Autodesk Inventor part; units mm, degrees
ref_plane "YZ Plane" through (0, 0, 0) normal (1, 0, 0) x (0, 1, 0)
ref_plane "XZ Plane" through (0, 0, 0) normal (0, 1, 0) x (-1, 0, 0)
ref_plane "XY Plane" through (0, 0, 0) normal (0, 0, 1) x (1, 0, 0)
sketch "スケッチ1" plane through (0, 0, 0) normal (0, 1, 0) x (-1, 0, 0)
  line L0 (0, 0) -> (-90, 0)
  line L1 (-90, 0) -> (-90, 50)
  line L2 (0, 50) -> (0, 0)
  line L3 (0, 0) -> (-5, 0)
  line L4 (-5, 0) -> (-5, 50)
  line L5 (-5, 0) -> (-90, 0)
  line L6 (-90, 0) -> (-85, 0)
  line L7 (-85, 0) -> (-85, 50)
  arc A0 (-85, 50) -> (-5, 50) centre (-45, 50) ccw
  line L8 (0, 0) -> (0, 10)
  line L9 (0, 10) -> (-90, 10)
  circle A1 centre (-45, 50) radius 45
  line L10 (-90, 5) -> (0, 5)
  line L11 (-90, 50) -> (-85, 50)
  line L12 (-5, 50) -> (0, 50)
  line L13 (0, 0) -> (-90, 0)
  line L14 (-90, 0) -> (-90, 5)
  line L15 (-90, 5) -> (0, 5)
  line L16 (0, 5) -> (0, 0)
  dimension "d0" = 90
  dimension "d1" = 50
  dimension "d2" = 5
  dimension "d3" = 85
  dimension "d4" = 5
  dimension "d5" = 80
  dimension "d6" = 10
  dimension "d7" = 90
extrude "押し出し1" add sketch "スケッチ1" along normal blind 230 contours L0 L4 L10 L2 | L0 L7 L10 L4 | L10 L4 L9 L2 | L0 L1 L10 L7 | L10 A1 L9 L4 | L9 L4 A1 L2 | L10 L1 L9 L7 | L7 L9 A1 L10 | L9 A1 L4 | A1 L9 | A1 L4 L12 | L9 L1 A1 L7 | L7 A1 L9 | A1 L9 A0 L4 | A1 L7 A0 L9 | L11 L7 A1
sketch "スケッチ2" plane through (0, 0, 0) normal (0, -1, 0) x (1, 0, 0)
  line L0 (0, 0) -> (0, 50)
  line L1 (90, 0) -> (0, 0)
  line L2 (90, 50) -> (90, 0)
  line L3 (85, 50) -> (90, 50)
  arc A0 (5, 50) -> (85, 50) centre (45, 50) ccw
  line L4 (0, 50) -> (5, 50)
  arc A1 (5, 23.467) -> (85, 23.467) centre (45, 50) ccw
  line L5 (0, 5) -> (90, 5)
  line L6 (5, 23.467) -> (5, 5)
  line L7 (85, 23.467) -> (85, 5)
  dimension "d29" = 48
extrude "押し出し2" cut sketch "スケッチ2" against normal blind 225 contours L6 A1 L5 | L5 A1 L7
sketch "スケッチ3" plane through (0, 230, 0) normal (0, 1, 0) x (1, 0, 0)
  arc A0 (85, -50) -> (5, -50) centre (45, -50) ccw
  line L0 (90, -50) -> (90, 0)
  line L1 (0, -50) -> (5, -50)
  arc A1 (85, -50) -> (5, -50) centre (45, -50) ccw
  line L2 (5, -50) -> (85, -50)
extrude "押し出し3" add sketch "スケッチ3" against normal blind 5
sketch "スケッチ4" plane through (90, 0, 50) normal (1, 0, 0) x (0, 0, -1)
  line L0 (0, 0) -> (50, 0)
  line L1 (0, 0) -> (0, 230)
  line L2 (25, 0) -> (25, 65)
  line L3 (25, 65) -> (25, 75)
  line L4 (25, 75) -> (25, 215)
  line L5 (25, 215) -> (25, 225)
  line L6 (0, 65) -> (40, 65)
  line L7 (40, 65) -> (40, 75)
  line L8 (40, 75) -> (0, 75)
  line L9 (0, 75) -> (0, 65)
  line L10 (0, 215) -> (40, 215)
  line L11 (40, 215) -> (40, 225)
  line L12 (40, 225) -> (0, 225)
  line L13 (0, 225) -> (0, 215)
  dimension "d16" = 65
  dimension "d17" = 10
  dimension "d18" = 140
  dimension "d19" = 10
  dimension "d20" = 40
extrude "押し出し4" cut sketch "スケッチ4" against normal blind 90 contours L1 L8 L3 L6 | L3 L8 L7 L6 | L1 L12 L5 L10 | L5 L12 L11 L10
sketch "スケッチ6" plane through (90, 0, 50) normal (1, 0, 0) x (0, 0, -1)
  line L0 (0, 230) -> (50, 230)
  line L1 (50, 230) -> (37.5, 251.6506)
  line L2 (50, 230) -> (110, 230) construction
  line L3 (0, 230) -> (37.5, 251.6506)
  line L4 (0, 230) -> (43.3013, 230) construction
  dimension "d32" = 120
  dimension "d33" = 30
extrude "押し出し6" add sketch "スケッチ6" against normal blind 90
sketch "スケッチ9" plane through (0, 0, 0) normal (-1, 0, 0) x (0, 0, 1)
  line L0 (10, 225) -> (50, 225)
  line L1 (50, 225) -> (50, 230)
  line L2 (50, 230) -> (12.5, 251.6506)
  line L3 (12.5, 251.6506) -> (0, 230)
  line L4 (0, 0) -> (0, 230)
  line L5 (0, 0) -> (50, 0)
  line L6 (50, 0) -> (50, 65)
  line L7 (50, 65) -> (10, 65)
  line L8 (10, 65) -> (10, 75)
  line L9 (10, 75) -> (50, 75)
  line L10 (50, 75) -> (50, 215)
  line L11 (50, 215) -> (10, 215)
  line L12 (10, 215) -> (10, 225)
  line L13 (12.5, 251.6506) -> (0, 230)
  line L14 (0, 230) -> (-132.7906, 0)
  line L15 (0, 145) -> (-49.0748, 145)
  line L16 (0, 115) -> (-66.3953, 115)
  dimension "d45" = 30
sketch "スケッチ10" plane through (0, 0, 0) normal (-1, 0, 0) x (0, 0, 1)
  line L0 (10, 225) -> (50, 225)
  line L1 (50, 225) -> (50, 230)
  line L2 (50, 230) -> (12.5, 251.6506)
  line L3 (12.5, 251.6506) -> (0, 230)
  line L4 (0, 0) -> (0, 230)
  line L5 (0, 0) -> (50, 0)
  line L6 (50, 0) -> (50, 65)
  line L7 (50, 65) -> (10, 65)
  line L8 (10, 65) -> (10, 75)
  line L9 (10, 75) -> (50, 75)
  line L10 (50, 75) -> (50, 215)
  line L11 (50, 215) -> (10, 215)
  line L12 (10, 215) -> (10, 225)
  line L13 (12.5, 251.6506) -> (-87.5, 78.4456)
  line L14 (-87.5, 78.4456) -> (50, 0)
sketch "スケッチ11" plane through (90, 230, 0) normal (0, 0.5, -0.866) x (-1, 0, 0)
  line L0 (0, 25) -> (90, 25)
  line L1 (45, 25) -> (45, 15)
  line L2 (45, 15) -> (60, 15)
  line L3 (60, 15) -> (30, 15)
  point P0 (90, -199.1858)
  dimension "d49" = 10
  dimension "d50" = 15
  dimension "d51" = 30
hole "穴1" at (45, 242.9904, 7.5) at (30, 242.9904, 7.5) at (60, 242.9904, 7.5) direction (0, -0.5, 0.866) diameter 2.5 depth 8 tip angle 118
sketch "スケッチ12" plane through (90, 0, 50) normal (1, 0, 0) x (0, 0, -1)
  line L0 (50, 0) -> (50, 230)
  line L1 (40, 225) -> (40, 215)
  line L2 (0, 215) -> (0, 75)
  line L3 (0, 145) -> (50, 145)
  line L4 (32.5, 175) -> (17.5, 175)
  line L5 (17.5, 175) -> (17.5, 115)
  line L6 (17.5, 115) -> (32.5, 115)
  line L7 (32.5, 115) -> (32.5, 175)
  line L8 (32.5, 175) -> (17.5, 115) construction
  line L9 (17.5, 175) -> (32.5, 115) construction
  line L10 (17.5, 145) -> (32.5, 145)
  line L11 (32.5, 145) -> (32.5, 115)
  line L12 (32.5, 115) -> (17.5, 115)
  line L13 (17.5, 115) -> (17.5, 145)
  point P0 (25, 145)
  dimension "d59" = 15
  dimension "d60" = 60
extrude "押し出し8" cut sketch "スケッチ12" against normal blind 2.5 contours L3 L7 L6 L5
sketch "スケッチ13" plane through (0, 0, 0) normal (-1, 0, 0) x (0, 0, 1)
  line L0 (0, 0) -> (0, 230)
  line L1 (50, 75) -> (50, 215)
  line L2 (50, 145) -> (0, 145)
  line L3 (17.5, 175) -> (32.5, 175)
  line L4 (32.5, 175) -> (32.5, 115)
  line L5 (32.5, 115) -> (17.5, 115)
  line L6 (17.5, 115) -> (17.5, 175)
  line L7 (17.5, 175) -> (32.5, 115) construction
  line L8 (32.5, 175) -> (17.5, 115) construction
  line L9 (17.5, 145) -> (32.5, 145)
  line L10 (32.5, 145) -> (32.5, 115)
  line L11 (32.5, 115) -> (17.5, 115)
  line L12 (17.5, 115) -> (17.5, 145)
  point P0 (25, 145)
  dimension "d63" = 15
  dimension "d64" = 60
extrude "押し出し9" cut sketch "スケッチ13" against normal blind 2.5 contours L4 L5 L6 L2
sketch "スケッチ14" plane through (90, 0, 0) normal (0, 0, -1) x (-1, 0, 0)
  line L0 (90, 0) -> (90, 230)
  line L1 (0, 0) -> (0, 230)
  line L2 (0, 145) -> (90, 145)
  line L3 (37.5, 175) -> (52.5, 175)
  line L4 (52.5, 175) -> (52.5, 115)
  line L5 (52.5, 115) -> (37.5, 115)
  line L6 (37.5, 115) -> (37.5, 175)
  line L7 (37.5, 175) -> (52.5, 115) construction
  line L8 (52.5, 175) -> (37.5, 115) construction
  line L9 (37.5, 145) -> (52.5, 145)
  line L10 (52.5, 145) -> (52.5, 175)
  line L11 (52.5, 175) -> (37.5, 175)
  line L12 (37.5, 175) -> (37.5, 145)
  point P0 (45, 145)
  dimension "d67" = 15
  dimension "d70" = 30
extrude "押し出し10" cut sketch "スケッチ14" against normal blind 2.5 contours L6 L3 L4 L2
sketch "スケッチ16" plane through (90, 0, 0) normal (0, 0, -1) x (-1, 0, 0)
  line L0 (52.5, 175) -> (52.5, 145)
  line L1 (52.5, 145) -> (37.5, 145)
  line L2 (37.5, 145) -> (37.5, 175)
  line L3 (90, 0) -> (90, 230)
  line L4 (0, 0) -> (0, 230)
  line L5 (0, 145) -> (90, 145)
  line L6 (0, 160) -> (37.5, 160)
  line L7 (52.5, 160) -> (90, 160)
  line L8 (18.75, 160) -> (18.75, 145)
  line L9 (71.25, 145) -> (71.25, 160)
  line L10 (11.25, 175) -> (26.25, 175)
  line L11 (26.25, 175) -> (26.25, 115)
  line L12 (26.25, 115) -> (11.25, 115)
  line L13 (11.25, 115) -> (11.25, 175)
  line L14 (11.25, 175) -> (26.25, 115) construction
  line L15 (26.25, 175) -> (11.25, 115) construction
  line L16 (11.25, 115) -> (26.25, 115)
  line L17 (26.25, 115) -> (26.25, 175)
  line L18 (26.25, 175) -> (11.25, 175)
  line L19 (11.25, 175) -> (11.25, 115)
  line L20 (45, 145) -> (45, 125)
  line L21 (78.75, 175) -> (63.75, 175)
  line L22 (63.75, 115) -> (78.75, 115)
  line L23 (78.75, 175) -> (78.75, 115)
  line L24 (63.75, 115) -> (63.75, 175)
  line L25 (63.75, 175) -> (78.75, 175)
  line L26 (78.75, 175) -> (78.75, 115)
  line L27 (78.75, 115) -> (63.75, 115)
  line L28 (63.75, 115) -> (63.75, 175)
  line L29 (11.25, 115) -> (26.25, 115)
  line L30 (26.25, 115) -> (26.25, 175)
  line L31 (26.25, 175) -> (11.25, 175)
  line L32 (11.25, 175) -> (11.25, 115)
  dimension "d71" = 15
  dimension "d72" = 60
  dimension "d73" = 20
extrude "押し出し11" cut sketch "スケッチ16" against normal blind 3 contours L24 L21 L23 L7 | L7 L9 L5 L24 | L5 L23 L22 L24 | L7 L23 L5 L9 | L11 L12 L13 L5 | L5 L8 L6 L11 | L6 L13 L10 L11 | L5 L13 L6 L8
sketch "スケッチ17" plane through (37.5, 145, 0) normal (0, 1, 0) x (1, 0, 0)
  line L0 (0, 0) -> (15, 0)
  line L1 (0, 0) -> (0, -2.5)
  line L2 (0, -2.5) -> (15, -2.5)
  line L3 (15, 0) -> (15, -2.5)
  line L4 (-57.7643, 16.522) -> (69.053, 16.522)
  line L5 (69.053, 16.522) -> (69.053, -65.9751)
  line L6 (69.053, -65.9751) -> (-57.7643, -65.9751)
  line L7 (-57.7643, -65.9751) -> (-57.7643, 16.522)
  point P0 (-37.5, 0)
properties part number "知能ロボコン発射台２．３" material "ABS プラスチック"
Design review of the part built by this model. Coordinates are the model's own, in mm. A direction names the side the tool comes from. Coordinates: 2 decimals unless noted, no trailing zeros. Order: outer loops, then holes, each group sorted by start corner. A loop starts at its lowest first (then second) coordinate and runs counter-clockwise, first axis right, second up.
Item 1: The part is to be moulded in two halves that separate along Y. For faces 5 (the flat face through (56, 0, 9)), 6 (the flat face through (44, 113, 0)), 7 (the flat face through (88, 220, 10)), say which applies: pulls with the +Y half, pulls with the -Y half, needs draft (parallel to the pull), parting line crosses it, or undercut.
Item 2: Take a section at B-B, the plane y = 71. Write out the cut boundary in (x, z), then the cut area to 3 significant figures.
Item 3: For line 1 (Y direction, x = 25, z = 12.5); line 2 (Y direction, x = 82, z = 22); line 3 (X direction, y = 152, z = 9), list the stretches that pass through material, from the lowest coordinate up.
Item 4: Take a section at C-C, the plane x = 67. Write out the cut boundary in (y, z), then the cut area to 3 significant figures.
Item 5: For pin 1 Ø12 at (x, z) = (27, 27) entering from +Y; pin 2 Ø1.5 at (x, y) = (87.5, 219.5) entering from +Z; pin 3 Ø1.5 at (x, y) = (68.5, 147.5) entering from +Z, all flat-tipped, find the tip position at first contact; note any pin that passes through.
Item 6: Take a section at A-A, the plane y = 104. Write out the cut boundary in (x, z).
Item 7: For faces 1 (the flat face through (87.5, 130, 25)), 2 (the cylindrical face through (44.16, 240.16, 10.55)), 3 (the flat face through (19, 145, 3)), 4 (the flat face through (9, 215, 24)), list the 3-axis set-ups (+Z, -Z, +X, -X, +Y, -Y) from which the entire face can be reached by the end or side of a thin tool; tool diameter is ignored.
The answers:
1. face 5: pulls with the -Y half
1. face 6: needs draft
1. face 7: undercut
2. outline: (0, 0) - (90, 0) - (90, 10) - (85, 10) - (85, 5) - (61.7, 5) arc R48 ccw to (71.53, 10) - (18.47, 10) arc R48 ccw to (28.3, 5) - (5, 5) - (5, 10) - (0, 10) - close
2. area: 721 mm2
3. line 1: y = 0 to 65, 75 to 215, 225 to 251.65
3. line 2: y = 0 to 65, 75 to 215, 225 to 246.17
3. line 3: x = 0 to 5, 20.04 to 69.96, 85 to 90
4. outline: (0, 0) - (115, 0) - (115, 3) - (175, 3) - (175, 0) - (230, 0) - (251.65, 12.5) - (230, 50) - (225, 50) - (225, 10) - (215, 10) - (215, 16.59) - (75, 16.59) - (75, 10) - (65, 10) - (65, 16.59) - (0, 16.59) - (0, 7.34) - (225, 7.34) - (225, 5) - (0, 5) - close
4. area: 3,690 mm2
5. pin 1: stops at y = 246.74
5. pin 2: stops at z = 10
5. pin 3: stops at z = 18.19
6. outline: (0, 0) - (90, 0) - (90, 50) - (85, 50) arc R40 cw to (5, 50) - (0, 50) - close; hole (5, 5) - (28.3, 5) arc R48 cw to (5, 23.47) - close; hole (61.7, 5) - (85, 5) - (85, 23.47) arc R48 cw to start
7. face 1: +X
7. face 2: none
7. face 3: -Z
7. face 4: +Z, +X, -X
